Geometry check sheet. Reference: the model listing, model coordinates, mm. A direction names the side the tool comes from. Coordinates: 2 decimals unless noted, no trailing zeros. Loops run counter-clockwise (first coordinate to the right, second up) from the corner with the lowest first, then second, coordinate; pieces in that order, holes last. Notation, with made-up numbers: (-27, 19.25) -> (28, 19.25) arc R26 cw to (28, 53.25) -> close; hole circle Ø2 at (79, -1). An arc over 180 degrees is marked (long way). Answer as a JSON object with one key per item and string values.
from build123d import *

# Parameters (mm, degrees)
EXTRUDE_1_DEPTH     = 5
SKETCH_4_W          = 40
SKETCH_4_H          = 8.5
CUT_EXTRUDE_1_DEPTH = 5
SKETCH_5_R          = 1.25
CUT_EXTRUDE_2_DEPTH = 7
SKETCH_9_R          = 6.5
CUT_EXTRUDE_4_DEPTH = 5
SKETCH_10_R         = 7.5
CUT_EXTRUDE_5_DEPTH = 1.1


with BuildPart() as part:
    # 草图3 → 凸台-拉伸1 (new body)
    with BuildSketch(Plane.XY):
        with BuildLine():
            Line((-35.723215038, 7.743839121), (-58.858024221, -11.158625231))
            ThreePointArc((-58.858024221, -11.158625231), (-60.178030432, -31.612892204), (-39.681768347, -31.462245799))
            Line((-39.681768347, -31.462245799), (-22.972363252, -13.241253001))
            ThreePointArc((-22.972363252, -13.241253001), (-19.627898346, -10.846108205), (-15.602197786, -10))
            Line((-15.602197786, -10), (15.602197786, -10))
            ThreePointArc((15.602197786, -10), (19.627898346, -10.846108205), (22.972363252, -13.241253001))
            Line((22.972363252, -13.241253001), (39.681768347, -31.462245799))
            ThreePointArc((39.681768347, -31.462245799), (60.178030432, -31.612892204), (58.858024221, -11.158625231))
            Line((58.858024221, -11.158625231), (35.723215038, 7.743839121))
            ThreePointArc((35.723215038, 7.743839121), (32.754745755, 9.419086771), (29.39605488, 10))
            Line((29.39605488, 10), (-29.39605488, 10))
            ThreePointArc((-29.39605488, 10), (-32.754745755, 9.419086771), (-35.723215038, 7.743839121))
        make_face()
    extrude(amount=EXTRUDE_1_DEPTH)

    # 草图4 → 切除-拉伸1 (cut)
    with BuildSketch(Plane.XY.offset(5)):
        with Locations((0, -0.75)):
            Rectangle(SKETCH_4_W, SKETCH_4_H)
    extrude(amount=-CUT_EXTRUDE_1_DEPTH, mode=Mode.SUBTRACT)

    # 草图5 → 切除-拉伸2 (cut)
    with BuildSketch(Plane.XY.offset(5)):
        with Locations((-29, -5)):
            Circle(SKETCH_5_R)
        with Locations((-29, 5)):
            Circle(SKETCH_5_R)
    cut_extrude_2 = extrude(amount=-CUT_EXTRUDE_2_DEPTH, mode=Mode.SUBTRACT)

    # 草图9 → 切除-拉伸4 (cut)
    with BuildSketch(Plane(origin=(0, 0, 0), x_dir=(-1, 0, 0), z_dir=(0, 0, -1))):
        with Locations((-50, -22)):
            Circle(SKETCH_9_R)
        with Locations((50, -22)):
            Circle(SKETCH_9_R)
    extrude(amount=-CUT_EXTRUDE_4_DEPTH, mode=Mode.SUBTRACT)

    # 草图10 → 切除-拉伸5 (cut)
    with BuildSketch(Plane(origin=(0, 0, 0), x_dir=(-1, 0, 0), z_dir=(0, 0, -1))):
        with Locations((-50, -22)):
            Circle(SKETCH_10_R)
        with Locations((50, -22)):
            Circle(SKETCH_10_R)
    extrude(amount=-CUT_EXTRUDE_5_DEPTH, mode=Mode.SUBTRACT)

    # 镜向1: 切除-拉伸2 across plane
    add(cut_extrude_2.mirror(Plane.ZY), mode=Mode.SUBTRACT)


solid = part.part
1. Mould release check, pull along X, two halves, no side actions. Record for faces 1 (the face through (-1, -8, 0)), 2 (the face through (0, 3.5, 3)), 3 (the face through (20, -1, 3)): released by +X, released by -X, zero draft, split by the parting line, or undercut.
Evaluation:
{"face 1": "zero draft", "face 2": "undercut", "face 3": "undercut"}
2. Section check D-D, the plane y = 0.5. Record the boundary of the cut face in (x, z), then the cut area to 3 significant figures.
Evaluation:
{"outline": "(-44.59, 0) -> (-20, 0) -> (-20, 5) -> (-44.59, 5) -> close; (20, 0) -> (44.59, 0) -> (44.59, 5) -> (20, 5) -> close", "area": "246 mm^2"}
3. Section check B-B, the plane z = 4.05. Record the boundary of the cut face in (x, y), then the cut area to 3 significant figures.
Evaluation:
{"outline": "(-58.86, -11.16) arc R14 ccw (long way) to (-39.68, -31.46) -> (-22.97, -13.24) arc R10 cw to (-15.6, -10) -> (15.6, -10) arc R10 cw to (22.97, -13.24) -> (39.68, -31.46) arc R14 ccw (long way) to (58.86, -11.16) -> (35.72, 7.74) arc R10 ccw to (29.4, 10) -> (-29.4, 10) arc R10 ccw to (-35.72, 7.74) -> close; hole circle Ø13 at (-50, -22); hole circle Ø2.5 at (-29, -5); hole circle Ø2.5 at (-29, 5); hole (-20, -5) -> (20, -5) -> (20, 3.5) -> (-20, 3.5) -> close; hole circle Ø2.5 at (29, -5); hole circle Ø2.5 at (29, 5); hole circle Ø13 at (50, -22)", "area": "2,710 mm^2"}
4. Depth check by flat-ended pin: P1, Ø2.5, axis at y = -2.5, z = 2.5, coming from the +X side; P2, Ø2.5, axis at x = 0, z = 2, coming from the -Y side; P3, Ø1.5, axis at x = -30.5, z = 4, coming from the -Y side. Enter the tip coordinate at first touch or a pass-through.
Evaluation:
{"P1": "stops at x = 49.79", "P2": "stops at y = -10", "P3": "stops at y = -22.27"}
5. Section check A-A, the plane x = -8.5. Record the boundary of the cut face in (y, z), then the cut area to 3 significant figures.
Evaluation:
{"outline": "(-10, 0) -> (-5, 0) -> (-5, 5) -> (-10, 5) -> close; (3.5, 0) -> (10, 0) -> (10, 5) -> (3.5, 5) -> close", "area": "57.5 mm^2"}
6. Tool access check on faces 4 (the face through (-20, -1, 3)), 5 (the face through (-44, -19, 1.1)), 6 (the face through (-19.68, -10.87, 2.46)). Record the directions out of +Z, -Z, +X, -X, +Y, -Y that give a thin tool (end or side, any length) a straight path to the whole face; none if there is none.
Evaluation:
{"face 4": "+Z, -Z", "face 5": "-Z", "face 6": "+Z, -Z, -Y"}
7. Thickness scan on probe 1 along Y at (x, z) = (-12, 4.05); probe 2 along X at (y, z) = (-24, 1.9); probe 3 along Y at (x, z) = (28, 1.4). Record the ranges inside material, lowest first. Write a range as from..to.
Evaluation:
{"probe 1": "y = -10..-5, 3.5..10", "probe 2": "x = -63.86..-56.18, -43.82..-32.84, 32.84..43.82, 56.18..63.86", "probe 3": "y = -18.72..-5.75, -4.25..4.25, 5.75..10"}
8. Section check C-C, the plane y = -22. Record the boundary of the cut face in (x, z), then the cut area to 3 significant figures.
Evaluation:
{"outline": "(-64, 0) -> (-57.5, 0) -> (-57.5, 1.1) -> (-56.5, 1.1) -> (-56.5, 5) -> (-64, 5) -> close; (-43.5, 1.1) -> (-42.5, 1.1) -> (-42.5, 0) -> (-31, 0) -> (-31, 5) -> (-43.5, 5) -> close; (31, 0) -> (42.5, 0) -> (42.5, 1.1) -> (43.5, 1.1) -> (43.5, 5) -> (31, 5) -> close; (56.5, 1.1) -> (57.5, 1.1) -> (57.5, 0) -> (64, 0) -> (64, 5) -> (56.5, 5) -> close", "area": "196 mm^2"}
